from build123d import *

# Parameters (mm, degrees)
SKETCH1_R               = 12.5
BOSS_EXTRUDE1_DEPTH     = 25.4
SKETCH2_R               = 9.9949
BOSS_EXTRUDE2_DEPTH     = 30
SKETCH4_R               = 15
BOSS_EXTRUDE3_DEPTH     = 10
SKETCH5_R               = 20
BOSS_EXTRUDE4_DEPTH     = 1
CUT_EXTRUDE1_DEPTH      = 1
CUT_EXTRUDE1_DEPTH_BACK = 56.4
CHAMFER1_SIZE           = 3


with BuildPart() as part:
    # Sketch1 → Boss-Extrude1 (new body)
    with BuildSketch(Plane.XY):
        Circle(SKETCH1_R)
    extrude(amount=BOSS_EXTRUDE1_DEPTH)

    # Sketch2 → Boss-Extrude2 (add)
    with BuildSketch(Plane.XY.offset(25.4)):
        Circle(SKETCH2_R)
    extrude(amount=BOSS_EXTRUDE2_DEPTH)

    # Sketch4 → Boss-Extrude3 (add)
    with BuildSketch(Plane.XY.offset(25.4)):
        Circle(SKETCH4_R)
        with BuildLine():
            ThreePointArc((-14.997117089, 0.294073132), (-14.892515339, 1.792480649), (-14.638580274, 3.272914233))
            Line((-14.638580274, 3.272914233), (-17.871018407, 2.150976779))
            Line((-17.871018407, 2.150976779), (-14.997117089, 0.294073132))
        make_face()
        with BuildLine():
            ThreePointArc((-14.730535341, -2.830429043), (-14.93975583, -1.343017399), (-14.999169305, 0.157861228))
            Line((-14.999169305, 0.157861228), (-17.927706996, -1.611620878))
            Line((-17.927706996, -1.611620878), (-14.730535341, -2.830429043))
        make_face()
        with BuildLine():
            ThreePointArc((-14.608252857, 3.4057229), (-14.194400465, 4.849638691), (-13.638215041, 6.24492518))
            Line((-13.638215041, 6.24492518), (-17.033280558, 5.819566429))
            Line((-17.033280558, 5.819566429), (-14.608252857, 3.4057229))
        make_face()
        with BuildLine():
            ThreePointArc((-13.580937876, 6.368526235), (-12.875922179, 7.694844251), (-12.041794367, 8.94400293))
            Line((-12.041794367, 8.94400293), (-15.451106615, 9.233813101))
            Line((-15.451106615, 9.233813101), (-13.580937876, 6.368526235))
        make_face()
        with BuildLine():
            ThreePointArc((-11.960070742, 9.052994413), (-10.994704308, 10.203748193), (-9.919089497, 11.252184835))
            Line((-9.919089497, 11.252184835), (-13.193645169, 12.244497832))
            Line((-13.193645169, 12.244497832), (-11.960070742, 9.052994413))
        make_face()
        with BuildLine():
            ThreePointArc((-9.816491125, 11.341803295), (-8.6329651, 12.266699376), (-7.362872818, 13.068592268))
            Line((-7.362872818, 13.068592268), (-10.35955812, 14.720039251))
            Line((-10.35955812, 14.720039251), (-9.816491125, 11.341803295))
        make_face()
        with BuildLine():
            ThreePointArc((-7.243883742, 13.134920949), (-5.893923892, 13.793536934), (-4.484863267, 14.313839509))
            Line((-4.484863267, 14.313839509), (-7.07270867, 16.552244321))
            Line((-7.07270867, 16.552244321), (-7.243883742, 13.134920949))
        make_face()
        with BuildLine():
            ThreePointArc((-4.354683879, 14.353979529), (-2.897289927, 14.71753074), (-1.41084367, 14.933503278))
            Line((-1.41084367, 14.933503278), (-3.476747913, 17.661036888))
            Line((-3.476747913, 17.661036888), (-4.354683879, 14.353979529))
        make_face()
        with BuildLine():
            Line((1.724836566, 14.900501294), (0.271163412, 17.997957395))
            Line((0.271163412, 17.997957395), (-1.275163434, 14.945700325))
            ThreePointArc((-1.275163434, 14.945700325), (0.22596951, 14.998297829), (1.724836566, 14.900501294))
        make_face()
        with BuildLine():
            Line((4.007223594, 17.548280801), (1.860087771, 14.8842223))
            ThreePointArc((1.860087771, 14.8842223), (3.339352995, 14.623567334), (4.785133167, 14.216275904))
            Line((4.785133167, 14.216275904), (4.007223594, 17.548280801))
        make_face()
        with BuildLine():
            Line((7.568148876, 16.331660129), (4.914044216, 14.172232338))
            ThreePointArc((4.914044216, 14.172232338), (6.30679073, 13.609716775), (7.636296486, 12.910731039))
            Line((7.636296486, 12.910731039), (7.568148876, 16.331660129))
        make_face()
        with BuildLine():
            Line((10.798309737, 14.401267542), (7.753233347, 12.840847817))
            ThreePointArc((7.753233347, 12.840847817), (8.998591447, 12.001056285), (10.153717007, 11.040925276))
            Line((10.153717007, 11.040925276), (10.798309737, 14.401267542))
        make_face()
        with BuildLine():
            Line((13.556532646, 11.841470459), (10.253568978, 10.948256629))
            ThreePointArc((10.253568978, 10.948256629), (11.297110538, 9.867892049), (12.227371371, 8.688578098))
            Line((12.227371371, 8.688578098), (13.556532646, 11.841470459))
        make_face()
        with BuildLine():
            Line((15.722270026, 8.764144294), (12.305774442, 8.577174091))
            ThreePointArc((12.305774442, 8.577174091), (13.101891689, 7.303453579), (13.766630933, 5.956498364))
            Line((13.766630933, 5.956498364), (15.722270026, 8.764144294))
        make_face()
        with BuildLine():
            Line((17.200868763, 5.303782969), (13.820158513, 5.831227887))
            ThreePointArc((13.820158513, 5.831227887), (14.334057303, 4.419819141), (14.704222663, 2.964091069))
            Line((14.704222663, 2.964091069), (17.200868763, 5.303782969))
        make_face()
        with BuildLine():
            Line((17.927706996, 1.611620878), (14.730535341, 2.830429043))
            ThreePointArc((14.730535341, 2.830429043), (14.932481879, 1.4216135), (15, 0))
            ThreePointArc((15, 0), (14.999792325, -0.078931707), (14.999169305, -0.157861228))
            Line((14.999169305, -0.157861228), (17.927706996, 1.611620878))
        make_face()
        with BuildLine():
            Line((17.871018407, -2.150976779), (14.997117089, -0.294073132))
            ThreePointArc((14.997117089, -0.294073132), (14.892515339, -1.792480649), (14.638580274, -3.272914233))
            Line((14.638580274, -3.272914233), (17.871018407, -2.150976779))
        make_face()
        with BuildLine():
            Line((17.033280558, -5.819566429), (14.608252857, -3.4057229))
            ThreePointArc((14.608252857, -3.4057229), (14.194400465, -4.849638691), (13.638215041, -6.24492518))
            Line((13.638215041, -6.24492518), (17.033280558, -5.819566429))
        make_face()
        with BuildLine():
            Line((15.451106615, -9.233813101), (13.580937876, -6.368526235))
            ThreePointArc((13.580937876, -6.368526235), (12.875922179, -7.694844251), (12.041794367, -8.94400293))
            Line((12.041794367, -8.94400293), (15.451106615, -9.233813101))
        make_face()
        with BuildLine():
            Line((13.193645169, -12.244497832), (11.960070742, -9.052994413))
            ThreePointArc((11.960070742, -9.052994413), (10.994704308, -10.203748193), (9.919089497, -11.252184835))
            Line((9.919089497, -11.252184835), (13.193645169, -12.244497832))
        make_face()
        with BuildLine():
            Line((10.35955812, -14.720039251), (9.816491125, -11.341803295))
            ThreePointArc((9.816491125, -11.341803295), (8.6329651, -12.266699376), (7.362872818, -13.068592268))
            Line((7.362872818, -13.068592268), (10.35955812, -14.720039251))
        make_face()
        with BuildLine():
            Line((7.07270867, -16.552244321), (7.243883742, -13.134920949))
            ThreePointArc((7.243883742, -13.134920949), (5.893923892, -13.793536934), (4.484863267, -14.313839509))
            Line((4.484863267, -14.313839509), (7.07270867, -16.552244321))
        make_face()
        with BuildLine():
            Line((3.476747913, -17.661036888), (4.354683879, -14.353979529))
            ThreePointArc((4.354683879, -14.353979529), (2.897289927, -14.71753074), (1.41084367, -14.933503278))
            Line((1.41084367, -14.933503278), (3.476747913, -17.661036888))
        make_face()
        with BuildLine():
            ThreePointArc((1.275163434, -14.945700325), (-0.22596951, -14.998297829), (-1.724836566, -14.900501294))
            Line((-1.724836566, -14.900501294), (-0.271163412, -17.997957395))
            Line((-0.271163412, -17.997957395), (1.275163434, -14.945700325))
        make_face()
        with BuildLine():
            ThreePointArc((-1.860087771, -14.8842223), (-3.339352995, -14.623567334), (-4.785133167, -14.216275904))
            Line((-4.785133167, -14.216275904), (-4.007223594, -17.548280801))
            Line((-4.007223594, -17.548280801), (-1.860087771, -14.8842223))
        make_face()
        with BuildLine():
            ThreePointArc((-4.914044216, -14.172232338), (-6.30679073, -13.609716775), (-7.636296486, -12.910731039))
            Line((-7.636296486, -12.910731039), (-7.568148876, -16.331660129))
            Line((-7.568148876, -16.331660129), (-4.914044216, -14.172232338))
        make_face()
        with BuildLine():
            ThreePointArc((-7.753233347, -12.840847817), (-8.998591447, -12.001056285), (-10.153717007, -11.040925276))
            Line((-10.153717007, -11.040925276), (-10.798309737, -14.401267542))
            Line((-10.798309737, -14.401267542), (-7.753233347, -12.840847817))
        make_face()
        with BuildLine():
            ThreePointArc((-10.253568978, -10.948256629), (-11.297110538, -9.867892049), (-12.227371371, -8.688578098))
            Line((-12.227371371, -8.688578098), (-13.556532646, -11.841470459))
            Line((-13.556532646, -11.841470459), (-10.253568978, -10.948256629))
        make_face()
        with BuildLine():
            ThreePointArc((-12.305774442, -8.577174091), (-13.101891689, -7.303453579), (-13.766630933, -5.956498364))
            Line((-13.766630933, -5.956498364), (-15.722270026, -8.764144294))
            Line((-15.722270026, -8.764144294), (-12.305774442, -8.577174091))
        make_face()
        with BuildLine():
            ThreePointArc((-13.820158513, -5.831227887), (-14.334057303, -4.419819141), (-14.704222663, -2.964091069))
            Line((-14.704222663, -2.964091069), (-17.200868763, -5.303782969))
            Line((-17.200868763, -5.303782969), (-13.820158513, -5.831227887))
        make_face()
    extrude(amount=BOSS_EXTRUDE3_DEPTH)

    # Sketch5 → Boss-Extrude4 (add)
    with BuildSketch(Plane.XY.offset(35.4)):
        Circle(SKETCH5_R)
    extrude(amount=-BOSS_EXTRUDE4_DEPTH)

    # Sketch3 → Cut-Extrude1 (cut, two sides)
    with BuildSketch(Plane(origin=(0, 0, 0), x_dir=(-1, 0, 0), z_dir=(0, 0, -1))) as cut_extrude1_sk:
        Polygon((1.896610387, 4.211437091), (-2.698906314, 3.748231322), (-4.595516701, -0.46320577), (-1.896610387, -4.211437091), (2.698906314, -3.748231322), (4.595516701, 0.46320577), align=None)
    extrude(amount=CUT_EXTRUDE1_DEPTH, mode=Mode.SUBTRACT)
    extrude(cut_extrude1_sk.sketch, amount=-CUT_EXTRUDE1_DEPTH_BACK, mode=Mode.SUBTRACT)

    # Chamfer1
    chamfer1_edges = [part.edges().sort_by_distance(p)[0] for p in [
        (-3.246063544, 2.337321431, 0),
        (-3.647211508, -1.642512776, 0),
        (-0.401147964, -3.979834206, 0),
        (3.246063544, -2.337321431, 0),
        (3.647211508, 1.642512776, 0),
        (0.401147964, 3.979834206, 0),
    ]]
    chamfer(chamfer1_edges, length=CHAMFER1_SIZE)


solid = part.part
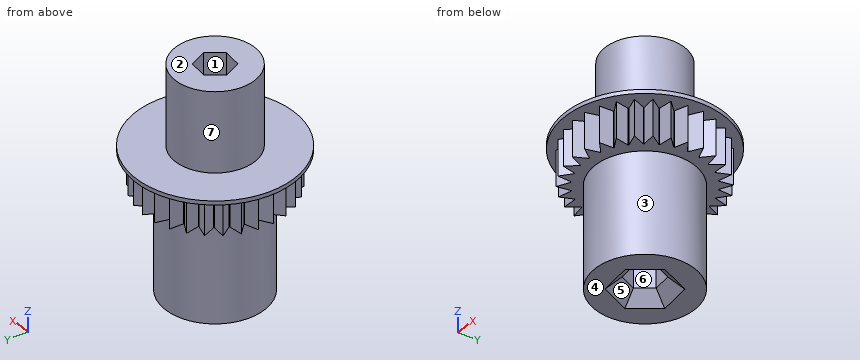
Part model, mm, in its own coordinate system. Face numbers are marked on the shaded views. A direction names the side the tool comes from. Round coordinates to 2 decimals unless told otherwise and drop trailing zeros. Write each loop counter-clockwise with the first axis right and the second up, starting at its lowest first coordinate (ties: lowest second). Pieces come first, ordered by that corner, then holes. Notation, with made-up numbers: (-22.75, 74.5) - (-2.75, 74.5) arc R24 ccw to (-2.75, 90.5) - close; hole circle Ø7 at (-23.75, -10). An arc over 180 degrees is marked (long way). Use CSV: the item, a comma, the result in double quotes.
Item 1: Slice it at C-C, the plane z = 39.5. Write the cut outline in (x, y), then the cut area to 3 significant figures.
Results list:
outline,"circle Ø19.99 at (0, 0); hole (-4.6, 0.46) - (-2.7, -3.75) - (1.9, -4.21) - (4.6, -0.46) - (2.7, 3.75) - (-1.9, 4.21) - close"
area,"258 mm²"
Item 2: Tool access for the marked faces 4, 5, 6 and 7: list every direction of +Z, -Z, +X, -X, +Y, -Y with a clear straight run to the whole face (end or side of a thin tool).
Results list:
face 4,"-Z, +X, -X, +Y, -Y"
face 5,"-Z"
face 6,"+Z, -Z"
face 7,"+Z"
Item 3: Pull direction Y, two halves, no side cores. Call the marked faces 1, 2 and 3: pulls with the +Y half, pulls with the -Y half, needs draft (parallel to the pull), parting line crosses it, or undercut.
Results list:
face 1,"undercut"
face 2,"needs draft"
face 3,"parting line crosses it"
Item 4: Flat gauge pins, fed straight in: P1, Ø5, axis at x = -15, y = -1.5, coming from the +Z side; P2, Ø3, axis at y = -6.5, z = 6, coming from the -X side; P3, Ø12, axis at x = -11, z = 12, coming from the -Y side. Where does each tip first touch, or does it go through?
Results list:
P1,"stops at z = 35.4"
P2,"stops at x = -11.46"
P3,"stops at y = -11.46"
Item 5: Slice it at B-B, the plane x = 6. Write the cut outline in (y, z), then the cut area to 3 significant figures.
Results list:
outline,"(-19.08, 34.4) - (-15.62, 34.4) - (-15.62, 25.4) - (-10.97, 25.4) - (-10.97, 0) - (-3.65, 0) - (-0.6, 1.78) - (3.72, 0) - (10.97, 0) - (10.97, 25.4) - (15.06, 25.4) - (15.06, 34.4) - (19.08, 34.4) - (19.08, 35.4) - (7.99, 35.4) - (7.99, 55.4) - (-7.99, 55.4) - (-7.99, 35.4) - (-19.08, 35.4) - close"
area,"1,180 mm²"
Item 6: Wall check: L1, parallel to Y at x = 16, z = 25.5; L2, parallel to Y at x = -7, z = 24.5; L3, parallel to Y at x = 0, z = 11. Give the ranges that are in metal, low to high.
Results list:
L1,"y = -5.95 to -4.79, -2.8 to -0.94, 0.45 to 2.35, 4.18 to 5.49"
L2,"y = -10.36 to 10.36"
L3,"y = -12.5 to -4.02, 4.02 to 12.5"
Item 7: Slice it at A-A, the plane z = 5. Write the cut outline in (x, y), then the cut area to 3 significant figures.
Results list:
outline,"circle Ø25 at (0, 0); hole (-4.6, 0.46) - (-2.7, -3.75) - (1.9, -4.21) - (4.6, -0.46) - (2.7, 3.75) - (-1.9, 4.21) - close"
area,"435 mm²"
